Work out the finished part from the listing and answer in its coordinate system (mm). A direction names the side the tool comes from. Give positions to 0.01 mm unless a question says otherwise; leave off trailing zeros. Write each loop counter-clockwise with the first axis right and the second up, starting at its lowest first coordinate (ties: lowest second). Pieces come first, ordered by that corner, then holes. Notation, with made-up numbers: (3.5, 23) -> (34.5, 23) arc R25 ccw to (34.5, 42) -> close; hole circle Ø7 at (89.25, 38). An arc over 180 degrees is marked (long way). Use a Markdown table: item, result. Add a question column.
Q1. Section A-A, the plane x = 0 is taken. Give the vertices of the cut face in (y, z) (3 decimals), plus the area to 3 significant figures.
Q2. Section C-C, the plane y = 17.5 is taken. Give the vertices of the cut face in (x, z).
Q3. Section B-B, the plane z = 0 is taken. Give the vertices of the cut face in (x, y) (3 decimals), plus the area to 3 significant figures.
Q4. Each of these flat-tipped pins is pushed along its axis until it touches: pin 1 Ø4 at (y, z) = (7, -5) entering from +X; pin 2 Ø1.5 at (x, y) = (4.5, 15.5) entering from +Z; pin 3 Ø2 at (x, y) = (-3.5, 3) entering from +Z. Where does it stop, or does it pass through?
Q5. For a pull along Z with two mould halves and no side action, classify faces 1 (the face through (0, 0, 7)), 2 (the face through (-1.409, 10.378, 6.345)), 3 (the face through (-1.604, 9.392, 7.224)) as pulls with the +Z half, pulls with the -Z half, needs draft (parallel to the pull), parting line crosses it, or undercut.
Q6. For faces 4 (the face through (3, 21.05, 6)), 5 (the face through (6.815, 20.036, -2.146)), determine the directions among +Z, -Z, +X, -X, +Y, -Y from which every point of the face is accessible in a straight line to the end or side of a thin tool.
Q7. Consider line 1 (Z direction, x = 0, y = 6); line 2 (Y direction, x = 5.75, z = 4.5). Determine where each line is inside the solid, lowest interval first.
from build123d import *

# Parameters (mm, degrees)
F0_R     = 7.4
F0_R_2   = 6.5
F1_DEPTH = 19.05
F2_R     = 7.145
F2_R_2   = 6.5
F3_DEPTH = 2
F5_ANGLE = -90


with BuildPart() as f1:
    # F0 (on Top) → F1 (new body)
    with BuildSketch(Plane.XY):
        Circle(F0_R)
        Circle(F0_R_2, mode=Mode.SUBTRACT)
    extrude(amount=F1_DEPTH)

    # F2 (on face) → F3 (join)
    with BuildSketch(Plane.XY.offset(19.05)):
        Circle(F2_R)
        Circle(F2_R_2, mode=Mode.SUBTRACT)
    extrude(amount=F3_DEPTH)


with BuildPart() as f1_1:
    # F5: moved
    add(f1.part.rotate(Axis((5.261217, 0, 0), (1, 0, 0)), F5_ANGLE))


solid = f1_1.part
Result set:
| question | item | result |
|---|---|---|
| 1 | outline | (0, -7.4) -> (19.05, -7.4) -> (19.05, -7.145) -> (21.05, -7.145) -> (21.05, -6.5) -> (0, -6.5) -> close; (0, 6.5) -> (21.05, 6.5) -> (21.05, 7.145) -> (19.05, 7.145) -> (19.05, 7.4) -> (0, 7.4) -> close |
| 1 | area | 36.9 mm2 |
| 2 | outline | circle Ø14.8 at (0, 0); hole circle Ø13 at (0, 0) |
| 3 | outline | (-7.4, 0) -> (-6.5, 0) -> (-6.5, 21.05) -> (-7.145, 21.05) -> (-7.145, 19.05) -> (-7.4, 19.05) -> close; (6.5, 0) -> (7.4, 0) -> (7.4, 19.05) -> (7.145, 19.05) -> (7.145, 21.05) -> (6.5, 21.05) -> close |
| 3 | area | 36.9 mm2 |
| 4 | pin 1 | stops at x = 6.76 |
| 4 | pin 2 | stops at z = 6.38 |
| 4 | pin 3 | stops at z = 6.96 |
| 5 | face 1 | needs draft |
| 5 | face 2 | undercut |
| 5 | face 3 | parting line crosses it |
| 6 | face 4 | +Z, -Z, +X, -X, +Y |
| 6 | face 5 | +Y |
| 7 | line 1 | z = -7.4 to -6.5, 6.5 to 7.4 |
| 7 | line 2 | y = 0 to 19.05 |
